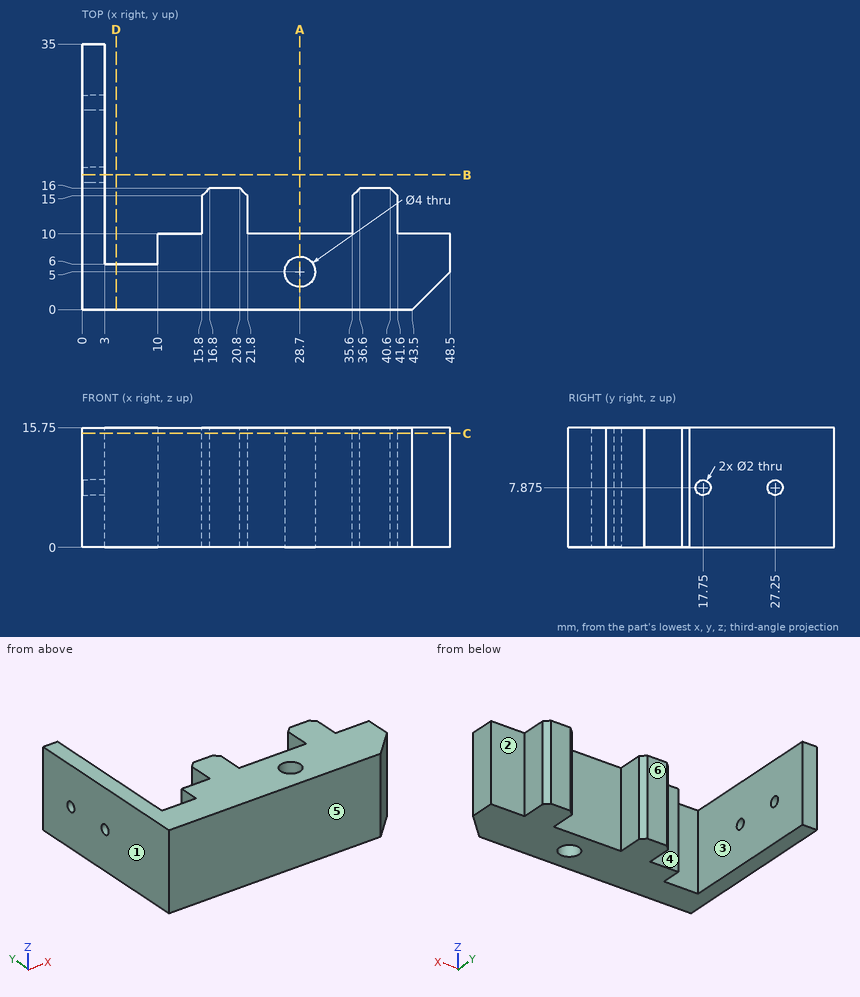
Study the drawing (mm; zero at the part's minimum x, y, z) and answer. A direction names the side the tool comes from. Coordinates: 2 decimals unless noted, no trailing zeros. Loops run counter-clockwise (first coordinate to the right, second up) from the corner with the lowest first, then second, coordinate; pieces in that order, holes last. Notation, with made-up numbers: (-12, -23) -> (-4, -23) arc R18 cw to (-4, 9) -> close; hole circle Ø11 at (89, 66.25). An arc over 180 degrees is marked (long way). Write item = value, one per line. Start each with the question number.
1) For the marked faces 4, 5 and 6, determine the directions among +Z, -Z, +X, -X, +Y, -Y from which every point of the face is accessible in a straight line to the end or side of a thin tool.
2) Find the intervals of material crossed by L1, parallel to X at y = 14.5, z = 13.5; L2, parallel to Z at x = 0.4, y = 27.25 (3 decimals); L3, parallel to X at y = 8, z = 7, in increasing order. Write a range as from..to.
3) The part is cut by section D-D, the plane x = 4.5. Determine the outline of the cut face in (y, z).
4) The part is cut by section C-C, the plane z = 15. Determine the outline of the cut face in (x, y), plus the area to 3 significant figures.
5) Given P1, Ø6, axis at y = 20.5, z = 5.5, coming from the -X side; P2, Ø3.5, axis at x = 43.5, z = 7.5, coming from the +Y side; P3, Ø5.5, axis at y = 13.5, z = 6.5, coming from the +X side; P4, Ø1.8, axis at y = 27.25, z = 7.875, coming from the +X side, each flat-ended and moving along its own axis, determine where each tip first touches the part or whether it passes through.
6) The mould has two halves that part along X. Classify the marked faces 1, 2 and 3: pulls with the +X half, pulls with the -X half, needs draft (parallel to the pull), parting line crosses it, or undercut.
7) The part is cut by section A-A, the plane x = 28.7. Determine the outline of the cut face in (y, z), plus the area to 3 significant figures.
8) The part is cut by section B-B, the plane y = 17.75. Determine the outline of the cut face in (x, z) (3 decimals), plus the area to 4 significant figures.
Result:
q1.face_4 = +Z, -Z, +Y
q1.face_5 = +Z, -Z, +X, -X, -Y
q1.face_6 = +Z, -Z, +X, +Y
q2.L1 = 0..3, 15.8..21.8, 35.6..41.6
q2.L2 = 0..6.875, 8.875..15.75
q2.L3 = 0..3, 10..48.5
q3.outline = (0, 0) -> (6, 0) -> (6, 15.75) -> (0, 15.75) -> close
q4.outline = (0, 0) -> (43.5, 0) -> (48.5, 5) -> (48.5, 10) -> (41.6, 10) -> (41.6, 15) -> (40.6, 16) -> (36.6, 16) -> (35.6, 15) -> (35.6, 10) -> (21.8, 10) -> (21.8, 15) -> (20.8, 16) -> (16.8, 16) -> (15.8, 15) -> (15.8, 10) -> (10, 10) -> (10, 6) -> (3, 6) -> (3, 35) -> (0, 35) -> close; hole circle Ø4 at (28.7, 5)
q4.area = 577 mm²
q5.P1 = 0
q5.P2 = 10
q5.P3 = 41.6
q5.P4 = through
q6.face_1 = pulls with the -X half
q6.face_2 = needs draft
q6.face_3 = undercut
q7.outline = (0, 0) -> (3, 0) -> (3, 15.75) -> (0, 15.75) -> close; (7, 0) -> (10, 0) -> (10, 15.75) -> (7, 15.75) -> close
q7.area = 94.5 mm²
q8.outline = (0, 0) -> (3, 0) -> (3, 6.875) -> (0, 6.875) -> close; (0, 8.875) -> (3, 8.875) -> (3, 15.75) -> (0, 15.75) -> close
q8.area = 41.25 mm²
